Part model, mm, in its own coordinate system. Face numbers are marked on the shaded views. Give positions to 0.01 mm unless a question says otherwise; leave off trailing zeros. Order: outer loops, then holes, each group sorted by start corner. A loop starts at its lowest first (then second) coordinate and runs counter-clockwise, first axis right, second up. Notation, with made-up numbers: M 36,-28.5 L 83,-28.5 A8 ccw 83,-19.5 Z; hole C 37,-39 d9. An arc over 180 degrees is marked long. Return JSON: item names as keys, results as strings.
from build123d import *

# Parameters (mm, degrees)
PIPE_TAP_DRILL_FOR_1_4_TAP1_D = 11.1252
F_1_4_CLEARANCE_HOLE1_D       = 6.7564
SKETCH7_R                     = 11.1125
BOSS_EXTRUDE1_DEPTH           = 6.35


with BuildPart() as part:
    # Sketch1 → Revolve1 (revolve)
    with BuildSketch(Plane.XY, mode=Mode.PRIVATE) as revolve1_sk:
        Polygon((0, 0), (47.498, 0), (47.498, 2.4638), (44.577, 2.4638), (44.577, 7.4422), (47.498, 7.4422), (47.498, 9.906), (41.148, 9.906), (41.148, 6.35), (0, 6.35), align=None)
    revolve(revolve1_sk.sketch.rotate(Axis((0, 48.192213231, 0), (0, -1, 0)), 180), axis=Axis((0, 48.192213231, 0), (0, -1, 0)))

    # Pipe Tap Drill for 1/4 Tap1 (through all)
    with Locations(Plane(origin=(0, 6.35, 0), x_dir=(1, 0, 0), z_dir=(0, 1, 0))):
        with Locations((0, 0), (-30.1752, 0)):
            Hole(PIPE_TAP_DRILL_FOR_1_4_TAP1_D / 2)

    # 1/4 Clearance Hole1 (through all)
    with Locations(Plane(origin=(0, 6.35, 0), x_dir=(1, 0, 0), z_dir=(0, 1, 0))):
        with Locations((12.150198978, 29.333175157), (-12.150198978, -29.333175157)):
            Hole(F_1_4_CLEARANCE_HOLE1_D / 2)

    # Sketch7 → Boss-Extrude1 (add)
    with BuildSketch(Plane(origin=(0, 6.35, 0), x_dir=(1, 0, 0), z_dir=(0, 1, 0))):
        Circle(SKETCH7_R)
    extrude(amount=-BOSS_EXTRUDE1_DEPTH)


solid = part.part
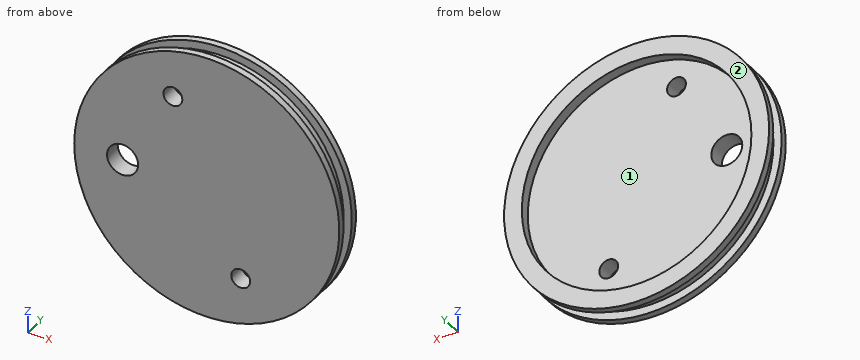
Q1. Pin check, flat tips, straight feed: pin 1 (5 mm diameter, centred on x = -17, z = -20.5, fed in from +Y); pin 2 (4 mm diameter, centred on x = 11, y = 6, fed in from +Z); pin 3 (1.5 mm diameter, centred on y = 6, z = 3, fed in from +X). Stop position of each tip, or through.
Established:
{"pin 1": "stops at y = 6.35", "pin 2": "stops at z = 46.51", "pin 3": "stops at x = 44.52"}
Q2. Band-saw the part on B-B (x = -31). Give the cut face in (y, z).
Established:
{"outline": "M 0,-35.99 L 2.46,-35.99 L 2.46,-32.03 L 7.44,-32.03 L 7.44,-35.99 L 9.91,-35.99 L 9.91,-27.06 L 6.35,-27.06 L 6.35,-5.5 L 0,-5.5 Z; M 0,5.5 L 6.35,5.5 L 6.35,27.06 L 9.91,27.06 L 9.91,35.99 L 7.44,35.99 L 7.44,32.03 L 2.46,32.03 L 2.46,35.99 L 0,35.99 Z"}
Q3. Two-plate mould, pull along X, no slides. Class the marked faces 1 and 2: +X half, -X half, draft (parallel to the pull), parting line (faces both ways), or undercut.
Established:
{"face 1": "undercut", "face 2": "draft"}
Q4. Probe line 1 along Z through (x, y) = (0, 7.9); line 2 along Y through (x, z) = (-29, 35.5); line 3 along Y through (x, z) = (34, -5.5). List the from-to ranges inside material, lowest first.
Established:
{"line 1": "z = -47.5 to -41.15, 41.15 to 47.5", "line 2": "y = 0 to 2.46, 7.44 to 9.91", "line 3": "y = 0 to 6.35"}
Q5. Band-saw the part on C-C (x = 0). Give the cut face in (y, z).
Established:
{"outline": "M 0,-47.5 L 2.46,-47.5 L 2.46,-44.58 L 7.44,-44.58 L 7.44,-47.5 L 9.91,-47.5 L 9.91,-41.15 L 6.35,-41.15 L 6.35,41.15 L 9.91,41.15 L 9.91,47.5 L 7.44,47.5 L 7.44,44.58 L 2.46,44.58 L 2.46,47.5 L 0,47.5 Z"}
Q6. Band-saw the part on D-D (z = -19). Give the cut face in (x, y).
Established:
{"outline": "M -43.53,0 L 43.53,0 L 43.53,2.46 L 40.33,2.46 L 40.33,7.44 L 43.53,7.44 L 43.53,9.91 L 36.5,9.91 L 36.5,6.35 L -36.5,6.35 L -36.5,9.91 L -43.53,9.91 L -43.53,7.44 L -40.33,7.44 L -40.33,2.46 L -43.53,2.46 Z"}
Q7. Band-saw the part on A-A (z = 0). Give the cut face in (x, y), then the cut area to 3 significant figures.
Established:
{"outline": "M -47.5,0 L -35.74,0 L -35.74,6.35 L -41.15,6.35 L -41.15,9.91 L -47.5,9.91 L -47.5,7.44 L -44.58,7.44 L -44.58,2.46 L -47.5,2.46 Z; M -24.61,0 L 47.5,0 L 47.5,2.46 L 44.58,2.46 L 44.58,7.44 L 47.5,7.44 L 47.5,9.91 L 41.15,9.91 L 41.15,6.35 L -24.61,6.35 Z", "area": "549 mm²"}
